Read the model definition and answer for the solid it produces. Units are mm, in the model's axes. A direction names the side the tool comes from. Coordinates: 2 decimals unless noted, no trailing zeros. Loops run counter-clockwise (first coordinate to the right, second up) from the corner with the lowest first, then second, coordinate; pieces in that order, holes last.
from build123d import *

# Parameters (mm, degrees)
SKETCH_R      = 16
PAD_DEPTH     = 5
SKETCH001_R   = 10
SKETCH001_R_2 = 5
PAD001_DEPTH  = 20
FILLET_R      = 3
CHAMFER_SIZE  = 2


with BuildPart() as part:
    # Sketch → Pad (new body)
    with BuildSketch(Plane.XY):
        Circle(SKETCH_R)
    extrude(amount=PAD_DEPTH)

    # Sketch001 (on Face3 of Pad) → Pad001 (join)
    with BuildSketch(Plane.XY.offset(5)):
        Circle(SKETCH001_R)
        Circle(SKETCH001_R_2, mode=Mode.SUBTRACT)
    extrude(amount=PAD001_DEPTH)

    # Fillet
    fillet_edges = [part.edges().sort_by_distance(p)[0] for p in [
        (-16, 0, 0),
    ]]
    fillet(fillet_edges, radius=FILLET_R)

    # Chamfer
    chamfer_edges = [part.edges().sort_by_distance(p)[0] for p in [
        (-10, 0, 25),
    ]]
    chamfer(chamfer_edges, length=CHAMFER_SIZE)


solid = part.part
Item 1: A cutting plane is placed at D-D on z = 4.5. Determine the outline of the cut face in (x, y), then the cut area to 3 significant figures.
Numbers:
outline: circle Ø32 at (0, 0)
area: 804 mm2
Item 2: Determine the mould class of faces 1 (the face through (-1.08, -4.88, 14.86)), 2 (the face through (5.2, 0.1, 25)), 3 (the face through (0, 0, 5)), 4 (the face through (-2.17, -9.76, 13.87)) for opening direction Y: released by +Y, released by -Y, zero draft, split by the parting line, or undercut.
Numbers:
face 1: undercut
face 2: zero draft
face 3: undercut
face 4: split by the parting line
Item 3: Given pin 1 (5 mm diameter, centred on y = -3, z = 19, fed in from -X); pin 2 (5 mm diameter, centred on x = -4.5, z = 12.5, fed in from -Y); pin 3 (2 mm diameter, centred on x = -8.5, z = 16, fed in from -Y); pin 4 (5 mm diameter, centred on x = -13, z = 13.5, fed in from +Y), each flat-ended and moving along its own axis, determine where each tip first touches the part or whether it passes through.
Numbers:
pin 1: stops at x = -9.99
pin 2: stops at y = -9.8
pin 3: stops at y = -6.61
pin 4: passes through
Item 4: A cutting plane is placed at C-C on z = 9.5. Determine the outline of the cut face in (x, y), then the cut area to 3 significant figures.
Numbers:
outline: circle Ø20 at (0, 0); hole circle Ø10 at (0, 0)
area: 236 mm2
Item 5: A cutting plane is placed at A-A on x = 0. Determine the outline of the cut face in (y, z).
Numbers:
outline: (-16, 3) arc R3 ccw to (-13, 0) - (13, 0) arc R3 ccw to (16, 3) - (16, 5) - (10, 5) - (10, 23) - (8, 25) - (5, 25) - (5, 5) - (-5, 5) - (-5, 25) - (-8, 25) - (-10, 23) - (-10, 5) - (-16, 5) - close
Item 6: Which of the six approach directions +Z, -Z, +X, -X, +Y, -Y give full straight-line access (tool end or side, diameter ignored) to faces 5 (the face through (10.4, 0.2, 5)), 6 (the face through (0, 0, 0))?
Numbers:
face 5: +Z
face 6: -Z, +X, -X, +Y, -Y
Item 7: Find the intervals of material crossed by line 1 along Y through (x, z) = (0, 19); line 2 along X through (y, z) = (-4.5, 16.5); line 3 along Z through (x, y) = (12, -0.5), in increasing order.
Numbers:
line 1: y = -10 to -5, 5 to 10
line 2: x = -8.93 to -2.18, 2.18 to 8.93
line 3: z = 0 to 5
